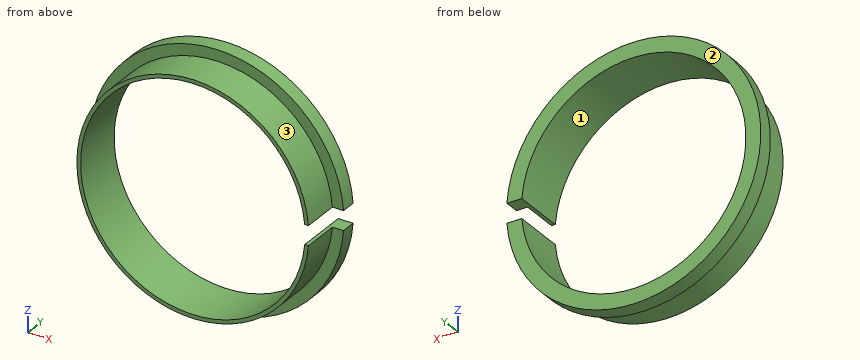
```python
from build123d import *

# Parameters (mm, degrees)
SKETCH1_R           = 15.5
SKETCH1_R_2         = 15
BOSS_EXTRUDE1_DEPTH = 7
BOSS_EXTRUDE2_START = -2
SKETCH2_R           = 16.99
SKETCH2_R_2         = 15.5
BOSS_EXTRUDE2_DEPTH = 2
SKETCH3_W           = 2.598251864
SKETCH3_H           = 7
CUT_EXTRUDE1_DEPTH  = 10


with BuildPart() as part:
    # Sketch1 → Boss-Extrude1 (new body)
    with BuildSketch(Plane(origin=(0, 0, 0), x_dir=(1, 0, 0), z_dir=(0, 1, 0))):
        with Locations(Location((0, 0, 0), (0, 0, 270))):
            Circle(SKETCH1_R)
        with Locations(Location((0, 0, 0), (0, 0, 270))):
            Circle(SKETCH1_R_2, mode=Mode.SUBTRACT)
    extrude(amount=BOSS_EXTRUDE1_DEPTH)

    # Sketch2 → Boss-Extrude2 (add)
    with BuildSketch(Plane(origin=(0, 7, 0), x_dir=(1, 0, 0), z_dir=(0, 1, 0)).offset(BOSS_EXTRUDE2_START)):
        with Locations(Location((0, 0, 0), (0, 0, 270))):
            Circle(SKETCH2_R)
        with Locations(Location((0, 0, 0), (0, 0, 270))):
            Circle(SKETCH2_R_2, mode=Mode.SUBTRACT)
    extrude(amount=BOSS_EXTRUDE2_DEPTH)

    # Sketch3 → Cut-Extrude1 (cut)
    with BuildSketch(Plane(origin=(16.99, 0, 0), x_dir=(0, 0, -1), z_dir=(1, 0, 0))):
        with Locations((0, 3.5)):
            Rectangle(SKETCH3_W, SKETCH3_H)
    extrude(amount=-CUT_EXTRUDE1_DEPTH, mode=Mode.SUBTRACT)


solid = part.part
```
Read the model definition and answer for the solid it produces. Units are mm, in the model's axes. Face numbers are marked on the shaded views. Give positions to 0.01 mm unless a question says otherwise; leave off trailing zeros. Order: outer loops, then holes, each group sorted by start corner. A loop starts at its lowest first (then second) coordinate and runs counter-clockwise, first axis right, second up. Notation, with made-up numbers: (1, 71.25) -> (16, 71.25) arc R23 cw to (16, 82.25) -> close; hole circle Ø10 at (62, 85.5). An arc over 180 degrees is marked (long way). One line per item, written item: value. Start each with the question number.
(1) The part is cut by section C-C (y = 2). Determine the outline of the cut face in (x, z).
(2) For a pull along Z with two mould halves and no side action, classify the marked faces 1, 2 and 3 as released by +Z, released by -Z, zero draft, split by the parting line, or undercut.
(3) The part is cut by section A-A (x = 0). Determine the outline of the cut face in (y, z).
(4) The part is cut by section D-D (y = 6). Determine the outline of the cut face in (x, z).
(5) Flat-ended cylindrical pins translate along their axes: P1, Ø2, axis at y = 3, z = -9.5, coming from the -X side; P2, Ø3, axis at x = -6, z = 13, coming from the -Y side; P3, Ø1.5, axis at y = 1.5, z = 6.5, coming from the -X side. Find the tip coordinate at first contact, or state that the pin passes through.
(6) The part is cut by section B-B (z = 3). Determine the outline of the cut face in (x, y), and give its area (3 significant figures).
(7) Straight lines are drawn through the part: L1, parallel to Z at x = 0, y = 4; L2, parallel to X at y = 5.25, z = 0; L3, parallel to Z at x = -10, y = 3.25. For each, find the intervals that lie inside material, in ascending order.
Taken from the geometry:
1. outline: (14.94, -1.3) arc R15 cw (long way) to (14.94, 1.3) -> (15.45, 1.3) arc R15.5 ccw (long way) to (15.45, -1.3) -> close
2. face 1: undercut
2. face 2: zero draft
2. face 3: split by the parting line
3. outline: (0, -15.5) -> (5, -15.5) -> (5, -16.99) -> (7, -16.99) -> (7, -15) -> (0, -15) -> close; (0, 15) -> (7, 15) -> (7, 16.99) -> (5, 16.99) -> (5, 15.5) -> (0, 15.5) -> close
4. outline: (14.94, -1.3) arc R15 cw (long way) to (14.94, 1.3) -> (16.94, 1.3) arc R16.99 ccw (long way) to (16.94, -1.3) -> close
5. P1: x = -12.96
5. P2: y = 0
5. P3: x = -14.39
6. outline: (-16.72, 5) -> (-15.21, 5) -> (-15.21, 0) -> (-14.7, 0) -> (-14.7, 7) -> (-16.72, 7) -> close; (14.7, 0) -> (15.21, 0) -> (15.21, 5) -> (16.72, 5) -> (16.72, 7) -> (14.7, 7) -> close
6. area: 13.2 mm^2
7. L1: -15.5 to -15, 15 to 15.5
7. L2: -16.99 to -15
7. L3: -11.84 to -11.18, 11.18 to 11.84
